from build123d import *

# Parameters (mm, degrees)
SKETCH1_W           = 5.9
SKETCH1_H           = 3.2
SKETCH1_W_2         = 4.9
SKETCH1_H_2         = 2.2
BOSS_EXTRUDE1_DEPTH = 1
SKETCH2_W           = 6.9
SKETCH2_H           = 4.2
SKETCH2_W_2         = 4.9
SKETCH2_H_2         = 2.2
BOSS_EXTRUDE2_DEPTH = 0.396875
SKETCH3_W           = 5.9
SKETCH3_H           = 3.2
SKETCH3_W_2         = 4.9
SKETCH3_H_2         = 2.2
BOSS_EXTRUDE3_DEPTH = 3


with BuildPart() as part:
    # Sketch1 → Boss-Extrude1 (new body)
    with BuildSketch(Plane.XY):
        with Locations((0, 5.4)):
            Rectangle(SKETCH1_W, SKETCH1_H)
        with Locations((0, 5.4)):
            Rectangle(SKETCH1_W_2, SKETCH1_H_2, mode=Mode.SUBTRACT)
    extrude(amount=BOSS_EXTRUDE1_DEPTH)

    # Sketch2 → Boss-Extrude2 (add)
    with BuildSketch(Plane.XY.offset(1)):
        with Locations((0, 5.4)):
            Rectangle(SKETCH2_W, SKETCH2_H)
        with Locations((0, 5.4)):
            Rectangle(SKETCH2_W_2, SKETCH2_H_2, mode=Mode.SUBTRACT)
    extrude(amount=BOSS_EXTRUDE2_DEPTH)

    # Sketch3 → Boss-Extrude3 (add)
    with BuildSketch(Plane.XY.offset(1.396875)):
        with Locations((0, 5.4)):
            Rectangle(SKETCH3_W, SKETCH3_H)
        with Locations((0, 5.4)):
            Rectangle(SKETCH3_W_2, SKETCH3_H_2, mode=Mode.SUBTRACT)
    extrude(amount=BOSS_EXTRUDE3_DEPTH)


solid = part.part
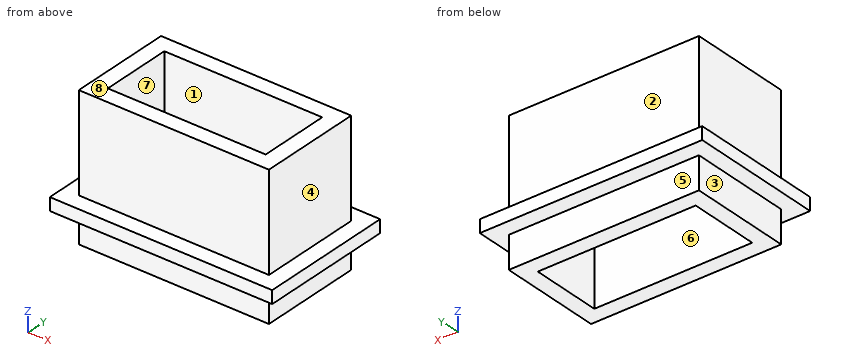
Work out the finished part from the listing and answer in its coordinate system (mm). Face numbers are marked on the shaded views. A direction names the side the tool comes from. Coordinates: 2 decimals unless noted, no trailing zeros. Write each loop counter-clockwise with the first axis right and the second up, starting at its lowest first coordinate (ties: lowest second). Pieces come first, ordered by that corner, then holes. Notation, with made-up numbers: M 43,60.5 L 70,60.5 A7 cw 70,71.5 Z; hole C -29.75,53.25 d3. An arc over 180 degrees is marked long. Use one line per item in the form item = value. Start each with the question number.
1. The part is cut by section A-A (x = 1). Give the vertices of the cut face in (y, z).
2. The part is cut by section B-B (y = 5.15). Give the vertices of the cut face in (x, z), plus the area to 3 significant figures.
3. The part is cut by section C-C (z = 2.1). Give the vertices of the cut face in (x, y), plus the area to 3 significant figures.
4. The mould has two halves that part along Y. Classify the marked faces 5, 6, 7 and 8: released by +Y, released by -Y, zero draft, split by the parting line, or undercut.
5. Straight lines are drawn through the part: probe 1 along X at (y, z) = (5.85, 1.45); probe 2 along Y at (x, z) = (1, 3.35); probe 3 along X at (y, z) = (5.5, 1.3). For each, find the intervals that lie inside material, in ascending order. Write a range as from..to.
6. Each of these flat-tipped pins is pushed along its axis until it touches: P1, Ø0.5, axis at x = 0, z = 0.5, coming from the +Y side; P2, Ø0.8, axis at y = 6, z = 0.5, coming from the -X side; P3, Ø0.5, axis at y = 5.5, z = 0.5, coming from the +X side. Where does it stop, or does it pass through?
7. A tool of negligible diameter and unlimited length cuts with its end or side. For the marked faces 1, 2, 3 and 4, from which of +Z, -Z, +X, -X, +Y, -Y can it reach the whole face along a straight path? Write none if from no direction.
Evaluation:
q1.outline = M 3.3,1 L 3.8,1 L 3.8,0 L 4.3,0 L 4.3,4.4 L 3.8,4.4 L 3.8,1.4 L 3.3,1.4 Z; M 6.5,0 L 7,0 L 7,1 L 7.5,1 L 7.5,1.4 L 7,1.4 L 7,4.4 L 6.5,4.4 Z
q2.outline = M -3.45,1 L -2.95,1 L -2.95,0 L -2.45,0 L -2.45,4.4 L -2.95,4.4 L -2.95,1.4 L -3.45,1.4 Z; M 2.45,0 L 2.95,0 L 2.95,1 L 3.45,1 L 3.45,1.4 L 2.95,1.4 L 2.95,4.4 L 2.45,4.4 Z
q2.area = 4.79 mm^2
q3.outline = M -2.95,3.8 L 2.95,3.8 L 2.95,7 L -2.95,7 Z; hole M -2.45,4.3 L 2.45,4.3 L 2.45,6.5 L -2.45,6.5 Z
q3.area = 8.10 mm^2
q4.face_5 = released by +Y
q4.face_6 = undercut
q4.face_7 = undercut
q4.face_8 = zero draft
q5.probe_1 = -2.95..-2.45, 2.45..2.95
q5.probe_2 = 3.8..4.3, 6.5..7
q5.probe_3 = -3.45..-2.45, 2.45..3.45
q6.P1 = 7
q6.P2 = -2.95
q6.P3 = 2.95
q7.face_1 = +Z, -Z
q7.face_2 = +Z, +X, -X, +Y
q7.face_3 = -Z, -X, +Y, -Y
q7.face_4 = +Z, +X, +Y, -Y
